Design review of the part shown in the three views and the two pictorial views. Dimensions are in mm from the part's minimum x, y and z. A direction names the side the tool comes from. Round coordinates to 2 decimals unless told otherwise and drop trailing zeros. Order: outer loops, then holes, each group sorted by start corner. A loop starts at its lowest first (then second) coordinate and runs counter-clockwise, first axis right, second up. Notation, with made-up numbers: (60, 21.5) - (106, 21.5) arc R18 ccw to (106, 41.5) - close; hole circle Ø3 at (3, 41.25). An arc over 180 degrees is marked (long way). One line per question, with ' | ' between items. Start each with the question number.
Item 1: Insertion check: pin 1 Ø5 at (x, y) = (4, 18.5) entering from +Z; pin 2 Ø3 at (x, z) = (3.5, 2) entering from +Y; pin 3 Ø5 at (y, z) = (16, 1.5) entering from +X; pin 4 Ø3.5 at (x, y) = (8.5, 17.5) entering from -Z. Each pin has a flat end and moves straight along its axis. Give the tip position at first contact, or say it passes through.
Item 2: Add section C-C on y = 16.75. State the section outline as (x, z) points.
Item 3: Tool access review of the marked faces 1, 2 and 3: name each direction out of +Z, -Z, +X, -X, +Y, -Y from which nothing blocks a thin tool from reaching the whole face with its end or side.
Item 4: Add section A-A on x = 4. State the section outline as (y, z) points.
Item 5: Draft analysis for pull direction Y (two halves, no side actions). For the marked faces 4, 5, 6 and 7, state which applies: +Y half, -Y half, draft (parallel to the pull), parting line (faces both ways), or undercut.
Item 6: Add section B-B on z = 6.75. State the section outline as (x, y) points.
Item 7: Add section D-D on x = 1.5. State the section outline as (y, z) points.
Item 8: For L1, parallel to Y at x = 8.5, z = 6.7; L2, parallel to Y at x = 4.25, z = 2.25; L3, parallel to Z at x = 7, y = 4.5, list the stretches that pass through material, from the lowest coordinate up. Write a range as [from, to].
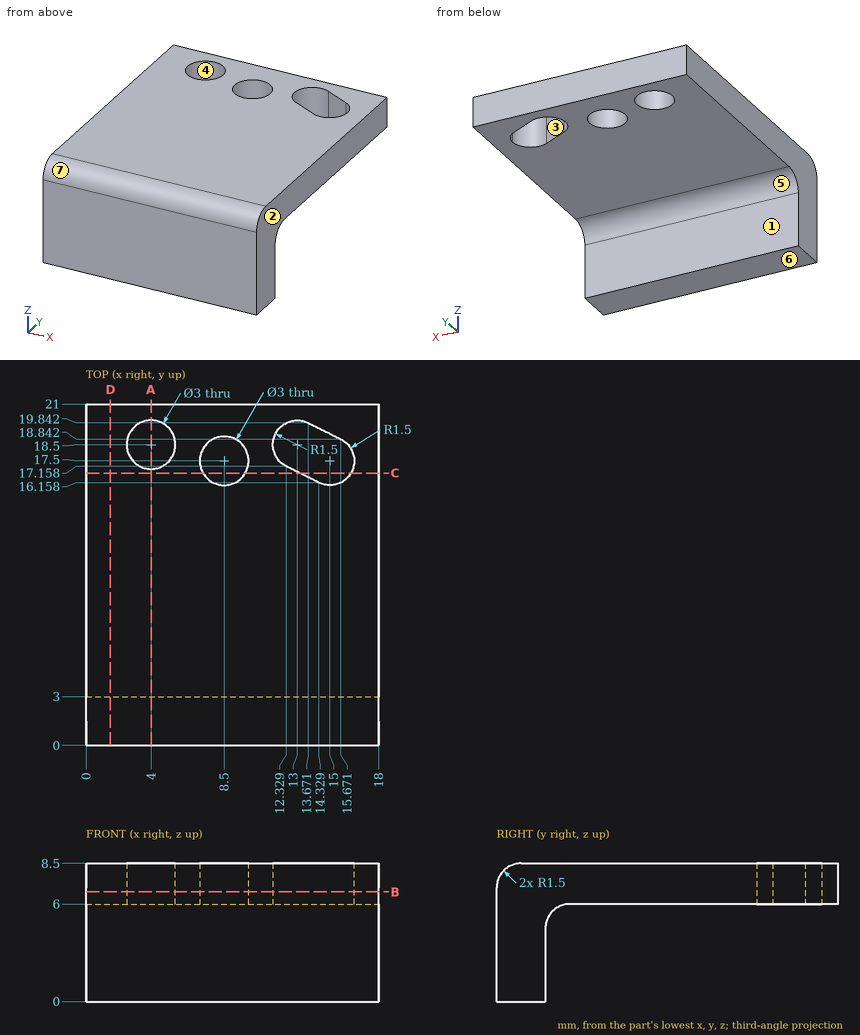
Determined:
1) pin 1: z = 8.5 | pin 2: y = 3 | pin 3: through | pin 4: z = 6
2) outline: (0, 6) - (7.2, 6) - (7.2, 8.5) - (0, 8.5) - close; (9.8, 6) - (13.15, 6) - (13.15, 8.5) - (9.8, 8.5) - close; (16.3, 6) - (18, 6) - (18, 8.5) - (16.3, 8.5) - close
3) face 1: -Z, +X, -X, +Y | face 2: +Z, -Z, +X, +Y, -Y | face 3: +Z, -Z
4) outline: (0, 0) - (3, 0) - (3, 4.5) arc R1.5 cw to (4.5, 6) - (17, 6) - (17, 8.5) - (1.5, 8.5) arc R1.5 ccw to (0, 7) - close; (20, 6) - (21, 6) - (21, 8.5) - (20, 8.5) - close
5) face 4: undercut | face 5: +Y half | face 6: draft | face 7: -Y half
6) outline: (0, 0) - (18, 0) - (18, 21) - (0, 21) - close; hole circle Ø3 at (4, 18.5); hole circle Ø3 at (8.5, 17.5); hole (12.33, 17.16) - (14.33, 16.16) arc R1.5 ccw to (15.67, 18.84) - (13.67, 19.84) arc R1.5 ccw to start
7) outline: (0, 0) - (3, 0) - (3, 4.5) arc R1.5 cw to (4.5, 6) - (21, 6) - (21, 8.5) - (1.5, 8.5) arc R1.5 ccw to (0, 7) - close
8) L1: [0, 16], [19, 21] | L2: [0, 3] | L3: [6, 8.5]
